from build123d import *

# Parameters (mm, degrees)
SKETCH_R        = 3.1
PAD_DEPTH       = 20
POCKET001_DEPTH = 10
SKETCH001_R     = 4.6
POCKET_DEPTH    = 3


with BuildPart() as part:
    # Sketch → Pad (new body, symmetric)
    with BuildSketch(Plane.XZ):
        with BuildLine():
            Line((-64, 8), (11, 8))
            ThreePointArc((12, 7), (11.707107, 7.707107), (11, 8))
            Line((12, 7), (12, 0))
            ThreePointArc((9.499513, -5.362311), (11.344155, -2.958328), (12, 0))
            ThreePointArc((1.937819, -9.996123), (5.890842, -7.960183), (9.499513, -5.362311))
            ThreePointArc((-8.966462, -11.52862), (-3.413443, -11.48016), (1.937819, -9.996123))
            ThreePointArc((-17.077228, -2.032133), (-14.868336, -8.357429), (-8.966462, -11.52862))
            Line((-16.97253, 0.96604), (-17.077228, -2.032133))
            ThreePointArc((-16.97253, 0.96604), (-17.237697, 1.679846), (-17.928591, 2))
            Line((-17.928591, 2), (-64.086659, 4.001878))
            ThreePointArc((-64, 8), (-65.99953, 6.04334), (-64.086659, 4.001878))
        make_face()
        Circle(SKETCH_R, mode=Mode.SUBTRACT)
    extrude(amount=PAD_DEPTH, both=True)

    # Sketch007 → Pocket001 (cut)
    with BuildSketch(Plane.XZ.offset(20)):
        with BuildLine():
            Line((12, 5.184354), (12, -34.815646))
            Line((12, -34.815646), (-17.928591, -34.815646))
            Line((-17.928591, 2), (-17.928591, -34.815646))
            ThreePointArc((0, 6.5), (-9.194185, 5.165908), (-17.928591, 2))
            ThreePointArc((12, 5.184354), (6.049918, 6.29748), (0, 6.5))
        make_face()
    pocket001 = extrude(amount=-POCKET001_DEPTH, mode=Mode.SUBTRACT)

    # Sketch001 → Pocket (cut)
    with BuildSketch(Plane.XZ.offset(10)):
        Circle(SKETCH001_R)
    pocket = extrude(amount=-POCKET_DEPTH, mode=Mode.SUBTRACT)

    # Mirrored: Pocket, Pocket001 across XZ
    add(pocket.mirror(Plane.XZ), mode=Mode.SUBTRACT)
    add(pocket001.mirror(Plane.XZ), mode=Mode.SUBTRACT)


solid = part.part
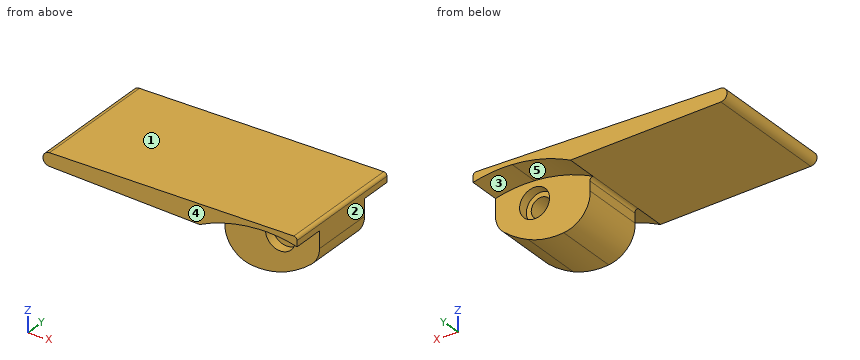
The model under review builds one solid part; all positions refer to its coordinate system, in mm. Face numbers are marked on the shaded views. A direction names the side the tool comes from. Round coordinates to 2 decimals unless told otherwise and drop trailing zeros. Write each loop counter-clockwise with the first axis right and the second up, starting at its lowest first coordinate (ties: lowest second). Pieces come first, ordered by that corner, then holes. Notation, with made-up numbers: (-16, 27.25) - (2, 27.25) arc R15 ccw to (2, 50.25) - close; hole circle Ø7 at (-33, -22). An arc over 180 degrees is marked (long way). One line per item, written item: value. Start each with the question number.
1. Clearance check with flat-ended pins moving along their axes: P1, Ø8, axis at x = -26.5, y = -8.5, coming from the -Z side; P2, Ø5.5, axis at x = -7.5, z = -7, coming from the -Y side; P3, Ø2, axis at x = -28, y = -12, coming from the -Z side. State where each tip first meets the part, or that it passes through.
2. The part is to be moulded in two halves that separate along X. For the marked faces 1, 2 and 3, say which applies: released by +X, released by -X, zero draft, split by the parting line, or undercut.
3. Consider section D-D on z = -8.25. Write out the cut boundary in (x, y), and give its area (3 significant figures).
4. Consider section A-A on y = 1.5. Write out the cut boundary in (x, z), and give its area (3 significant figures).
5. Consider section B-B on y = -16. Write out the cut boundary in (x, z), and give its area (3 significant figures).
6. To check wall thickness, follow L1, parallel to Z at x = 0, y = 0.25; L2, parallel to Y at x = 7.5, z = -0.75; L3, parallel to Y at x = 3.5, z = 2.25. State the ranges of each line that lie inside material, in increasing order. Write a range as from..to.
7. Consider section C-C on x = -11. Write out the cut boundary in (y, z), and give its area (3 significant figures).
8. Machinability: for the marked faces 4 and 5, which of the approach directions +Z, -Z, +X, -X, +Y, -Y give a long, thin tool a straight path to every point of the face, cutting with its end or side? Answer none if there is none.
Checks:
1. P1: stops at z = 2.2
1. P2: stops at y = -10
1. P3: stops at z = 2.39
2. face 1: zero draft
2. face 2: released by +X
2. face 3: undercut
3. outline: (-14.96, -10) - (5.41, -10) - (5.41, 10) - (-14.96, 10) - close
3. area: 407 mm^2
4. outline: (-64.09, 4) - (-17.93, 2) arc R1 cw to (-16.97, 0.97) - (-17.08, -2.03) arc R9.24 ccw to (-8.97, -11.53) arc R21.27 ccw to (1.94, -10) arc R30 ccw to (9.5, -5.36) arc R7 ccw to (12, 0) - (12, 7) arc R1 ccw to (11, 8) - (-64, 8) arc R2 ccw to start; hole circle Ø6.2 at (0, 0)
4. area: 712 mm^2
5. outline: (-64.09, 4) - (-17.93, 2) arc R45.7 cw to (0, 6.5) arc R40 cw to (12, 5.18) - (12, 7) arc R1 ccw to (11, 8) - (-64, 8) arc R2 ccw to start
5. area: 314 mm^2
6. L1: z = -10.71..-3.1, 3.1..8
6. L2: y = -10..10
6. L3: y = -7..7
7. outline: (-20, 4.67) - (-10, 4.67) - (-10, -11.04) - (10, -11.04) - (10, 4.67) - (20, 4.67) - (20, 8) - (-20, 8) - close
7. area: 447 mm^2
8. face 4: +Z, -Z, +X, -X, -Y
8. face 5: -Z, +Y
